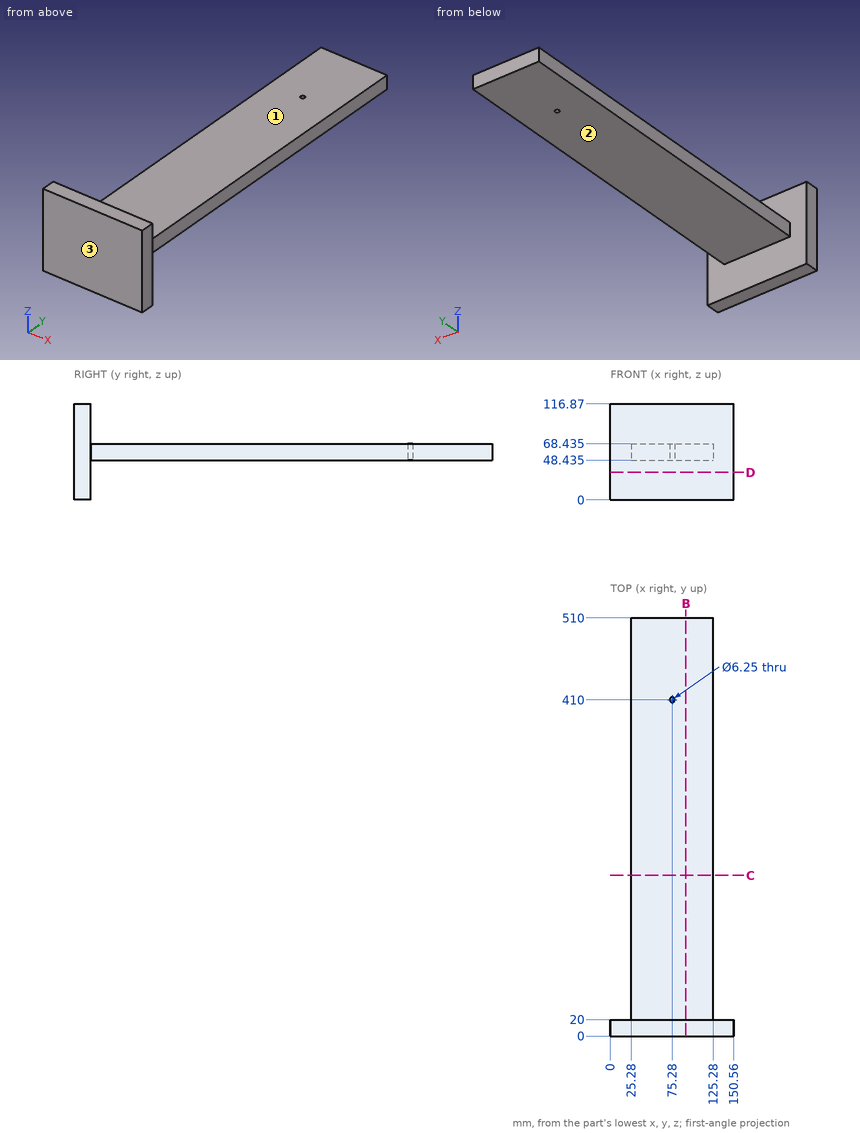
Answer from the drawing. Dimensions are ordinates in mm from the lowest x, y and z of the part. A direction names the side the tool comes from. Round coordinates to 2 decimals unless told otherwise and drop trailing zeros. Order: outer loops, then holes, each group sorted by start corner. A loop starts at its lowest first (then second) coordinate and runs counter-clockwise, first axis right, second up. Notation, with made-up numbers: (68, -9.5) -> (123, -9.5) arc R32 ccw to (123, 29.5) -> close; hole circle Ø9 at (46.25, 47.5). An arc over 180 degrees is marked (long way). Answer as CSV lines item,"result".
Q1. A cutting plane is placed at D-D on z = 33.5. Determine the outline of the cut face in (x, y), plus the area to 3 significant figures.
Computed values:
outline,"(0, 0) -> (150.56, 0) -> (150.56, 20) -> (0, 20) -> close"
area,"3,010 mm^2"
Q2. Consider line 1 (Y direction, x = 13, z = 14); line 2 (X direction, y = 410, z = 60.75) (1 decimal); line 3 (X direction, y = 106.5, z = 67). Determine where each line is inside the solid, lowest interval first. Write a range as from..to.
Computed values:
line 1,"y = 0..20"
line 2,"x = 25.3..72.2, 78.4..125.3"
line 3,"x = 25.28..125.28"
Q3. A cutting plane is placed at C-C on y = 196. Determine the outline of the cut face in (x, z) (1 decimal).
Computed values:
outline,"(25.3, 48.4) -> (125.3, 48.4) -> (125.3, 68.4) -> (25.3, 68.4) -> close"
Q4. A cutting plane is placed at B-B on x = 92. Determine the outline of the cut face in (y, z) (1 decimal), plus the area to 3 significant figures.
Computed values:
outline,"(0, 0) -> (20, 0) -> (20, 48.4) -> (510, 48.4) -> (510, 68.4) -> (20, 68.4) -> (20, 116.9) -> (0, 116.9) -> close"
area,"12,100 mm^2"
Q5. Given pin 1 (10 mm diameter, centred on x = 28, z = 89.5, fed in from +Y); pin 2 (10 mm diameter, centred on x = 60, y = 213, fed in from -Z) (1 decimal); pin 3 (16 mm diameter, centred on y = 304.5, z = 57, fed in from +X), each flat-ended and moving along its own axis, determine where each tip first touches the part or whether it passes through.
Computed values:
pin 1,"stops at y = 20"
pin 2,"stops at z = 48.4"
pin 3,"stops at x = 125.28"
Q6. Which of the six approach directions +Z, -Z, +X, -X, +Y, -Y give full straight-line access (tool end or side, diameter ignored) to the marked faces 1, 2 and 3?
Computed values:
face 1,"+Z, +X, -X, +Y"
face 2,"-Z, +X, -X, +Y"
face 3,"+Z, -Z, +X, -X, -Y"
